Could you check a few things on this model? Use its own coordinates, in mm. Face numbers are marked on the shaded views. A direction names the side the tool comes from. Round coordinates to 2 decimals unless told otherwise and drop trailing zeros. Order: outer loops, then holes, each group sorted by start corner. A loop starts at its lowest first (then second) coordinate and runs counter-clockwise, first axis right, second up. Notation, with made-up numbers: (-8, 21) - (14, 21) arc R25 cw to (14, 35) - close; hole circle Ø10 at (75.25, -22.5). An arc over 180 degrees is marked (long way). Return JSON: item names as keys, results as strings. Group by question number.
from build123d import *

# Parameters (mm, degrees)
F0_R     = 11.0109
F1_DEPTH = 6.35
F2_R     = 5.08
F3_R     = 5.08
F4_R     = 5.08
F5_R     = 5.08
F6_R     = 5.08
F7_R     = 5.08


with BuildPart() as f1:
    # F0 (on Top) → F1 (new body)
    with BuildSketch(Plane.XY):
        Polygon((7.417982, -12.848321), (14.835964, 0), (7.417982, 12.848321), (-7.417982, 12.848321), (-14.835964, 0), (-7.417982, -12.848321), align=None)
        Circle(F0_R, mode=Mode.SUBTRACT)
        with BuildLine():
            ThreePointArc((20.6375, -35.745199), (35.745199, -20.6375), (41.275, 0))
            Line((41.275, 0), (14.835964, 0))
            Line((14.835964, 0), (7.417982, -12.848321))
            Line((7.417982, -12.848321), (20.6375, -35.745199))
        make_face()
        with Locations((21.997045, -12.7)):
            Circle(F0_R, mode=Mode.SUBTRACT)
        with BuildLine():
            ThreePointArc((-41.275, 0), (-35.440503, -21.156474), (-19.586502, -36.331729))
            Line((-19.586502, -36.331729), (-7.417982, -12.848321))
            Line((-7.417982, -12.848321), (-14.835964, 0))
            Line((-14.835964, 0), (-41.275, 0))
        make_face()
        with Locations((-21.997045, -12.7)):
            Circle(F0_R, mode=Mode.SUBTRACT)
        with BuildLine():
            Line((7.417982, 12.848321), (20.6375, 35.745199))
            ThreePointArc((20.6375, 35.745199), (0, 41.275), (-20.6375, 35.745199))
            Line((-20.6375, 35.745199), (-7.417982, 12.848321))
            Line((-7.417982, 12.848321), (7.417982, 12.848321))
        make_face()
        with Locations((0, 25.4)):
            Circle(F0_R, mode=Mode.SUBTRACT)
    extrude(amount=F1_DEPTH)

    # F2
    f2_edges = [f1.edges().sort_by_distance(p)[0] for p in [
        (-19.586502, -36.331729, 3.175),
    ]]
    fillet(f2_edges, radius=F2_R)

    # F3
    f3_edges = [f1.edges().sort_by_distance(p)[0] for p in [
        (20.6375, -35.745199, 3.175),
    ]]
    fillet(f3_edges, radius=F3_R)

    # F4
    f4_edges = [f1.edges().sort_by_distance(p)[0] for p in [
        (-41.275, 0, 3.175),
    ]]
    fillet(f4_edges, radius=F4_R)

    # F5
    f5_edges = [f1.edges().sort_by_distance(p)[0] for p in [
        (-20.6375, 35.745199, 3.175),
    ]]
    fillet(f5_edges, radius=F5_R)

    # F6
    f6_edges = [f1.edges().sort_by_distance(p)[0] for p in [
        (41.275, 0, 3.175),
    ]]
    fillet(f6_edges, radius=F6_R)

    # F7
    f7_edges = [f1.edges().sort_by_distance(p)[0] for p in [
        (20.6375, 35.745199, 3.175),
    ]]
    fillet(f7_edges, radius=F7_R)


solid = f1.part
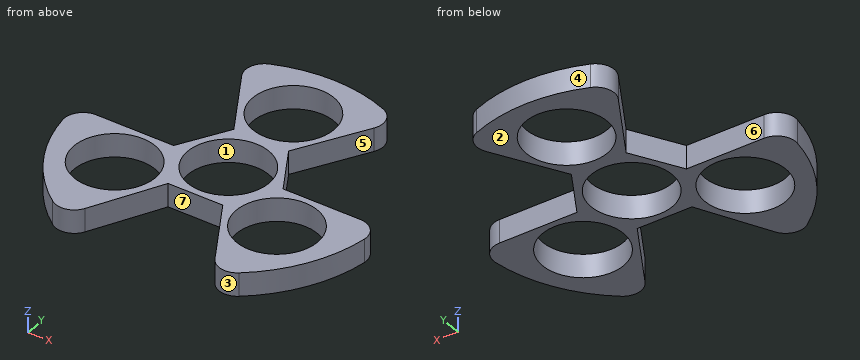
1) I want a section at C-C, the plane x = 30. List the corners of the cut face in (y, z) for me.
2) We'd pull the mould along Y, two halves only. Please class the marked faces 1, 2, 3 and 4: +Y half, -Y half, draft (parallel to the pull), parting line (faces both ways), or undercut.
3) I want a section at D-D, the plane y = -4. List the corners of the cut face in (x, z) for me, plus the area to 3 significant figures.
4) For the marked faces 5, 6 and 7, which set-ups out of +Z, -Z, +X, -X, +Y, -Y let a thin tool reach every point of the face, with its end or its side?
5) I want a section at A-A, the plane z = 3. List the corners of the cut face in (x, y) for me (3 decimals), plus the area to 3 significant figures.
6) I want a section at B-B, the plane y = 33. List the corners of the cut face in (x, z) for me.
7) Will these pins go through, and if not, where does the flat tip stop? pin 1 (3 mm diameter, centred on x = 14.5, z = 1, fed in from -Y); pin 2 (3 mm diameter, centred on x = 28.5, z = 4.5, fed in from +Y); pin 3 (3 mm diameter, centred on x = -30.5, z = 3, fed in from -Y).
8) If I drill on line 1 along Y through (x, z) = (22, 1.5); line 2 along Y through (x, z) = (4.5, 4.5); line 3 along X through (y, z) = (-19, 4), over which ranges is the centre line in solid material (lowest first)? Write a range as from..to.
Outcome:
{
 "1": {"outline": "(-28.35, 0) - (-20.26, 0) - (-20.26, 6.35) - (-28.35, 6.35) - close; (-5.14, 0) - (0, 0) - (0, 6.35) - (-5.14, 6.35) - close"},
 "2": {"face 1": "undercut", "face 2": "draft", "face 3": "-Y half", "face 4": "+Y half"},
 "3": {"outline": "(-40.8, 0) - (-28.75, 0) - (-28.75, 6.35) - (-40.8, 6.35) - close; (-15.25, 0) - (-10.26, 0) - (-10.26, 6.35) - (-15.25, 6.35) - close; (10.26, 0) - (15.25, 0) - (15.25, 6.35) - (10.26, 6.35) - close; (28.75, 0) - (40.8, 0) - (40.8, 6.35) - (28.75, 6.35) - close", "area": "216 mm^2"},
 "4": {"face 5": "+Z, -Z, +X", "face 6": "+Z, -Z, -X", "face 7": "+Z, -Z, -Y"},
 "5": {"outline": "(-40.866, -5.793) arc R41.275 ccw to (-24.575, -33.162) arc R5.08 ccw to (-17.04, -31.417) - (-7.418, -12.848) - (7.418, -12.848) - (17.918, -31.036) arc R5.08 ccw to (25.45, -32.495) arc R41.275 ccw to (40.866, -5.793) arc R5.08 ccw to (35.837, 0) - (14.836, 0) - (7.418, 12.848) - (17.918, 31.036) arc R5.08 ccw to (15.416, 38.288) arc R41.275 ccw to (-15.416, 38.288) arc R5.08 ccw to (-17.918, 31.036) - (-7.418, 12.848) - (-14.836, 0) - (-35.837, 0) arc R5.08 ccw to start; hole circle Ø22.022 at (-21.997, -12.7); hole circle Ø22.022 at (0, 0); hole circle Ø22.022 at (0, 25.4); hole circle Ø22.022 at (21.997, -12.7)", "area": "1,410 mm^2"},
 "6": {"outline": "(-18.57, 0) - (-7.97, 0) - (-7.97, 6.35) - (-18.57, 6.35) - close; (7.97, 0) - (18.57, 0) - (18.57, 6.35) - (7.97, 6.35) - close"},
 "7": {"pin 1": "y = -27.71", "pin 2": "y = 0", "pin 3": "y = -29.37"},
 "8": {"line 1": "-33.57..-23.71, -1.69..0", "line 2": "-12.85..-10.05, 10.05..15.35, 35.45..41.03", "line 3": "-36.64..-31.03, -12.97..-10.61, 10.97..12.97, 31.03..36.64"}
}
